Verification items for this drawing (mm, ordinates from the low corner). A direction names the side the tool comes from. Round coordinates to 2 decimals unless told otherwise and drop trailing zeros. Loops run counter-clockwise (first coordinate to the right, second up) from the corner with the lowest first, then second, coordinate; pieces in that order, holes last. Notation, with made-up numbers: (68, 48) -> (110, 48) arc R16 ccw to (110, 67) -> close; hole circle Ø4 at (50, 19). An arc over 180 degrees is marked (long way). One line per item, written item: value. Start each with the question number.
1. Cross-section at A-A on z = 2.25. Record the cut outline in (x, y) (1 decimal), then the cut area to 3 significant figures.
2. Set-up check for the marked faces 1 and 2: record each of +Z, -Z, +X, -X, +Y, -Y from which the full face is reachable in a straight line by a thin tool's end or side.
3. Material ranges on L1, parallel to Z at x = 7, y = 1.5; L2, parallel to Y at x = 6, z = 23.5 (1 decimal); L3, parallel to X at y = 7.5, z = 10.25 (1 decimal), recorded low to high.
4. Cross-section at D-D on z = 15.5. Record the cut outline in (x, y).
5. Cross-section at C-C on y = 5.25. Record the cut outline in (x, z) (1 decimal).
6. Go/stop test with flat-tipped pins: pin 1 (2 mm diameter, centred on y = 8, z = 20, fed in from +X); pin 2 (6 mm diameter, centred on y = 1, z = 3, fed in from +X) (1 decimal); pin 3 (3 mm diameter, centred on x = 8, y = 4, fed in from -Z); pin 4 (1 mm diameter, centred on y = 9.5, z = 3.5, fed in from +X). Record where each tip stops, or that it passes through.
7. Cross-section at B-B on x = 3.75. Record the cut outline in (y, z) (1 decimal).
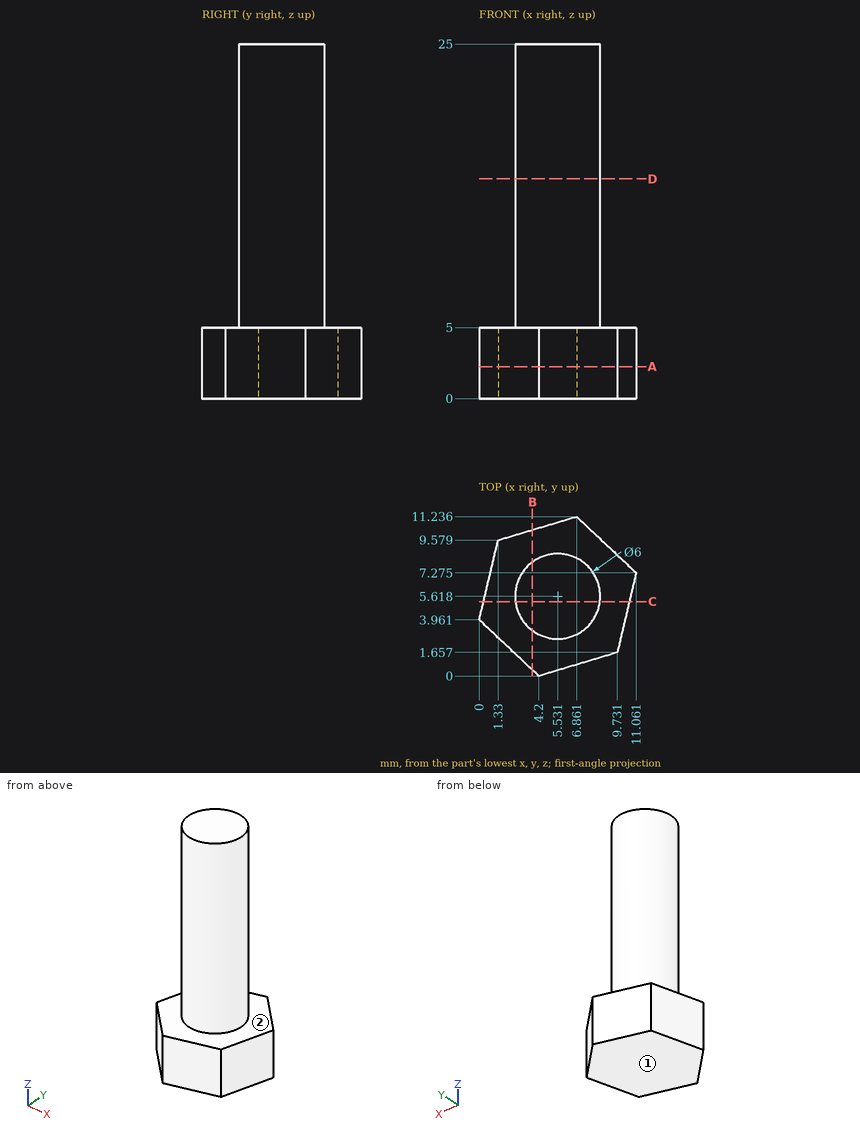
Taken from the geometry:
1. outline: (0, 4) -> (4.2, 0) -> (9.7, 1.7) -> (11.1, 7.3) -> (6.9, 11.2) -> (1.3, 9.6) -> close
1. area: 86.6 mm2
2. face 1: -Z, +X, -X, +Y, -Y
2. face 2: +Z
3. L1: z = 0 to 5
3. L2: y = 2.7 to 8.6
3. L3: x = 3.2 to 7.9
4. outline: circle Ø6 at (5.53, 5.62)
5. outline: (0.3, 0) -> (10.6, 0) -> (10.6, 5) -> (8.5, 5) -> (8.5, 25) -> (2.6, 25) -> (2.6, 5) -> (0.3, 5) -> close
6. pin 1: stops at x = 8.19
6. pin 2: stops at x = 10.3
6. pin 3: stops at z = 0
6. pin 4: stops at x = 9.23
7. outline: (0.4, 0) -> (10.3, 0) -> (10.3, 5) -> (8, 5) -> (8, 25) -> (3.2, 25) -> (3.2, 5) -> (0.4, 5) -> close
